```python
from build123d import *

# Parameters (mm, degrees)
FURO_COM_FOLGA_DE_M51_D = 5.5


with BuildPart() as part:
    # Esboço1 → Revolução1 (revolve)
    with BuildSketch(Plane.XY, mode=Mode.PRIVATE) as revolu_o1_sk:
        Polygon((17.5, 0), (17.5, 6), (31, 6), (31, 16), (35, 16), (35, 6), (45, 6), (45, 0), align=None)
    revolve(revolu_o1_sk.sketch.rotate(Axis((0, 0, 0), (0, 1, 0)), 90), axis=Axis((0, 0, 0), (0, 1, 0)))

    # Furo com folga de M51 (through all)
    with Locations(Plane(origin=(0, 6, 0), x_dir=(1, 0, 0), z_dir=(0, 1, 0))):
        with Locations((0, 40), (40, 0), (0, -40), (-40, 0)):
            Hole(FURO_COM_FOLGA_DE_M51_D / 2)


solid = part.part
```
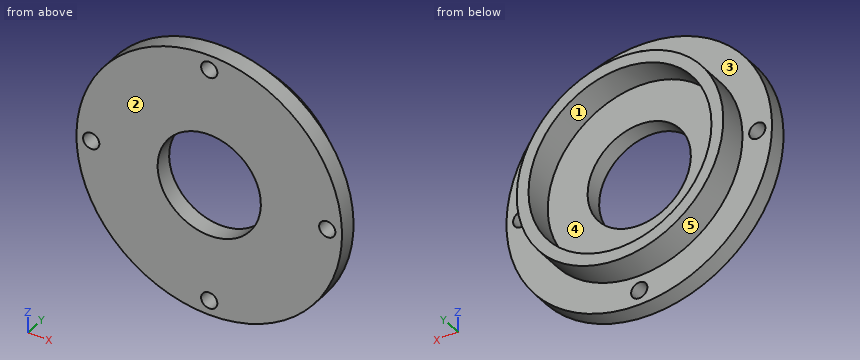
Build history of the part. All positions in model axes, mm. Face numbers are marked on the shaded views. A direction names the side the tool comes from. Round coordinates to 2 decimals unless told otherwise and drop trailing zeros. Order: outer loops, then holes, each group sorted by start corner. A loop starts at its lowest first (then second) coordinate and runs counter-clockwise, first axis right, second up. Notation, with made-up numbers: (29.25, 73) - (87.25, 73) arc R27 ccw to (87.25, 108) - close; hole circle Ø5 at (87.25, 72). An arc over 180 degrees is marked (long way). Use a Markdown table: item, result.
1) Saw through at D-D on z = -40. Write the cut outline in (x, y), and give its area (3 significant figures).
Recorded:
| item | result |
|---|---|
| outline | (-20.62, 0) - (-2.75, 0) - (-2.75, 6) - (-20.62, 6) - close; (2.75, 0) - (20.62, 0) - (20.62, 6) - (2.75, 6) - close |
| area | 214 mm² |
2) Tool access for the marked faces 1 and 2: list every direction of +Z, -Z, +X, -X, +Y, -Y with a clear straight run to the whole face (end or side of a thin tool).
Recorded:
| item | result |
|---|---|
| face 1 | +Y |
| face 2 | +Z, -Z, +X, -X, -Y |
3) Saw through at C-C on x = -40. Write the cut outline in (y, z).
Recorded:
| item | result |
|---|---|
| outline | (0, -20.62) - (6, -20.62) - (6, -2.75) - (0, -2.75) - close; (0, 2.75) - (6, 2.75) - (6, 20.62) - (0, 20.62) - close |
4) Wall check: L1, parallel to Y at x = 13, z = 23; L2, parallel to Z at x = -27.5, y = 9.25; L3, parallel to Z at x = 40, y = 3.95. Give the ranges that are in metal, low to high.
Recorded:
| item | result |
|---|---|
| L1 | y = 0 to 6 |
| L2 | z = -21.65 to -14.31, 14.31 to 21.65 |
| L3 | z = -20.62 to -2.75, 2.75 to 20.62 |
5) Saw through at A-A on z = 0. Write the cut outline in (x, y).
Recorded:
| item | result |
|---|---|
| outline | (-45, 0) - (-42.75, 0) - (-42.75, 6) - (-45, 6) - close; (-37.25, 0) - (-17.5, 0) - (-17.5, 6) - (-31, 6) - (-31, 16) - (-35, 16) - (-35, 6) - (-37.25, 6) - close; (17.5, 0) - (37.25, 0) - (37.25, 6) - (35, 6) - (35, 16) - (31, 16) - (31, 6) - (17.5, 6) - close; (42.75, 0) - (45, 0) - (45, 6) - (42.75, 6) - close |
6) Pull direction X, two halves, no side cores. Call the marked faces 3, 4 and 5: pulls with the +X half, pulls with the -X half, needs draft (parallel to the pull), parting line crosses it, or undercut.
Recorded:
| item | result |
|---|---|
| face 3 | needs draft |
| face 4 | undercut |
| face 5 | parting line crosses it |
7) Saw through at B-B on x = 0. Write the cut outline in (y, z), and give its area (3 significant figures).
Recorded:
| item | result |
|---|---|
| outline | (0, -45) - (6, -45) - (6, -42.75) - (0, -42.75) - close; (0, -37.25) - (6, -37.25) - (6, -35) - (16, -35) - (16, -31) - (6, -31) - (6, -17.5) - (0, -17.5) - close; (0, 17.5) - (6, 17.5) - (6, 31) - (16, 31) - (16, 35) - (6, 35) - (6, 37.25) - (0, 37.25) - close; (0, 42.75) - (6, 42.75) - (6, 45) - (0, 45) - close |
| area | 344 mm² |
8) Flat gauge pins, fed straight in: pin 1 Ø8 at (y, z) = (13.5, -16.5) entering from -X; pin 2 Ø5 at (x, y) = (9.5, 12.5) entering from +Z; pin 3 Ø5 at (y, z) = (10.5, -30.5) entering from +X; pin 4 Ø1.5 at (x, z) = (-25.5, -7) entering from -Y. Where does each tip first touch, or does it go through?
Recorded:
| item | result |
|---|---|
| pin 1 | stops at x = -32.69 |
| pin 2 | stops at z = 34.29 |
| pin 3 | stops at x = 21 |
| pin 4 | stops at y = 0 |
